Here's how the part is built. I have some questions about the finished solid (model axes, mm). A direction names the side the tool comes from. Coordinates: 2 decimals unless noted, no trailing zeros. Write each loop counter-clockwise with the first axis right and the second up, starting at its lowest first coordinate (ties: lowest second). Pieces come first, ordered by that corner, then holes. Notation, with made-up numbers: (-5, -33.75) -> (37, -33.75) arc R25 cw to (37, -12.75) -> close; hole circle Ø9 at (53, 67.5). An arc over 180 degrees is marked (long way). Put each result on its own line as item: value. Start each with the question number.
Item 1: For pin 1 (12 mm diameter, centred on x = -24, z = -40.5, fed in from +Y); pin 2 (5 mm diameter, centred on x = -10.5, z = -44.5, fed in from +Y); pin 3 (3 mm diameter, centred on y = -13, z = -85.5, fed in from +X); pin 4 (3.5 mm diameter, centred on x = 10.5, z = -44.5, fed in from +Y), each with a flat end and sliding along its axis, tell me the tip position at first contact or that it passes through.
Item 2: On a 3-axis mill with a long thin cutter (end or side, diameter ignored), from which of +Z, -Z, +X, -X, +Y, -Y can I reach the whole of each face in a straight line? I mean faces 1 (the face through (37, 20, -38)), 2 (the face through (0, -18, -52)), 3 (the face through (-50, 4.25, -20)), 4 (the face through (43.802, -2.095, -20.218)), 5 (the face through (-44.753, -0.121, -13.944)). Say none if no direction works.
Item 3: I want a section at C-C, the plane x = -47.5. List the corners of the cut face in (y, z) for me.
Item 4: I want a section at B-B, the plane x = -10.5. List the corners of the cut face in (y, z) for me.
Item 5: I want a section at D-D, the plane z = -126.5. List the corners of the cut face in (x, y) for me.
Item 6: I need wall thicknesses on line 1 (X direction, y = 0, z = -14.5); line 2 (X direction, y = 9, z = -44); line 3 (Z direction, x = -10.5, y = -5). Which ranges of each line are inside material? Lowest first, please. Write a range as [from, to].
Item 7: I want a section at A-A, the plane y = -13. List the corners of the cut face in (x, z) for me.
Item 8: If we mould it in two halves opening along Y, with no side actions, what happens to faces 6 (the face through (-36, 20, -38)), 7 (the face through (49, 0, -22.5)), 8 (the face through (37, -20, -38))? For each: released by +Y, released by -Y, zero draft, split by the parting line, or undercut.
from build123d import *

# Parameters (mm, degrees)
PAD_DEPTH       = 20
SKETCH003_R     = 2.2
HOLE_DEPTH      = 40.001
POCKET001_DEPTH = 4.5
SKETCH007_R     = 2.75
HOLE001_DEPTH   = 12
PAD001_DEPTH    = 101
SKETCH011_R     = 45
HOLE002_DEPTH   = 12
CHAMFER_SIZE    = 0.99
SKETCH009_W     = 35
SKETCH009_H     = 67.5
POCKET_DEPTH    = 2


with BuildPart() as part:
    # Sketch → Pad (new body, symmetric)
    with BuildSketch(Plane.XZ):
        with BuildLine():
            ThreePointArc((13.9194109071, -37.5), (29.6992968462, -26.794621976), (38.7298334621, -10))
            Line((38.7298334621, -10), (55, -10))
            Line((55, -10), (55, -45.8493649054))
            Line((0, -77.6036297108), (55, -45.8493649054))
            Line((-55, -45.8493649054), (0, -77.6036297108))
            Line((-55, -45.8493649054), (-55, -10))
            Line((-55, -10), (-38.7298334621, -10))
            ThreePointArc((-38.7298334621, -10), (-29.6992968462, -26.794621976), (-13.9194109071, -37.5))
            Line((-13.9194109071, -37.5), (13.9194109071, -37.5))
        make_face()
    extrude(amount=PAD_DEPTH, both=True)

    # Sketch003 → Hole (cut, through all)
    with BuildSketch(Plane.XZ.offset(20)):
        with Locations((-10.5, -44.5)):
            Circle(SKETCH003_R)
        with Locations((10.5, -44.5)):
            Circle(SKETCH003_R)
        with Locations((-10.5, -60.5)):
            Circle(SKETCH003_R)
        with Locations((10.5, -60.5)):
            Circle(SKETCH003_R)
    extrude(amount=-HOLE_DEPTH, mode=Mode.SUBTRACT)

    # Sketch006 → Pocket001 (cut)
    with BuildSketch(Plane(origin=(0, 0, -18), x_dir=(-1, 0, 0), z_dir=(0, 0, 1))):
        Polygon((55, 4.25), (45.0462616441, 4.25), (42.592523, 0), (45.0462616441, -4.25), (55, -4.25), align=None)
        Polygon((-55, 4.25), (-55, -4.25), (-45.0462616441, -4.25), (-42.592523, 0), (-45.0462616441, 4.25), align=None)
    extrude(amount=-POCKET001_DEPTH, mode=Mode.SUBTRACT)

    # Sketch007 (on Face5 of Pocket001) → Hole001 (cut)
    with BuildSketch(Plane(origin=(0, 0, -10), x_dir=(-1, 0, 0), z_dir=(0, 0, 1))):
        with Locations((47.5, 0)):
            Circle(SKETCH007_R)
        with Locations((-47.5, 0)):
            Circle(SKETCH007_R)
    extrude(amount=-HOLE001_DEPTH, mode=Mode.SUBTRACT)

    # Sketch010 (on Face10 of Hole001) → Pad001 (join)
    with BuildSketch(Plane(origin=(33.1033573777, 0, -57.3366968793), x_dir=(0.8660254038, 0, 0.5), z_dir=(0.5, 0, -0.8660254038))):
        Polygon((-38.8, 9), (-38.8, -9), (-26.8, -21), (-20.8, -21), (-2.8, -3), (-2.8, 3), (-20.8, 21), (-26.8, 21), align=None)
    extrude(amount=PAD001_DEPTH)

    # Sketch011 (on Face30 of Pad001) → Hole002 (cut)
    with BuildSketch(Plane(origin=(-33.6017856668, 0, -19.4), x_dir=(0.5, 0, -0.8660254038), z_dir=(-0.8660254038, 0, -0.5))):
        with Locations((117.5, 0)):
            Circle(SKETCH011_R)
    extrude(amount=-HOLE002_DEPTH, mode=Mode.SUBTRACT)

    # Chamfer
    chamfer_edges = [part.edges().sort_by_distance(p)[0] for p in [
        (9.460864, 20.5, -70.986697),
        (12.491953, 21, -69.236697),
        (15.523042, 20.5, -67.486697),
        (15.523042, -20.5, -67.486697),
        (12.491953, -21, -69.236697),
        (9.460864, -20.5, -70.986697),
    ]]
    chamfer(chamfer_edges, length=CHAMFER_SIZE)

    # Sketch009 → Pocket (cut)
    with BuildSketch(Plane(origin=(0, 20, 0), x_dir=(1, 0, 0), z_dir=(0, 1, 0))):
        with Locations((0, 33.75)):
            Rectangle(SKETCH009_W, SKETCH009_H)
    pocket = extrude(amount=-POCKET_DEPTH, mode=Mode.SUBTRACT)

    # Mirrored: Pocket across XZ
    add(pocket.mirror(Plane.XZ), mode=Mode.SUBTRACT)


solid = part.part
Calculated:
1. pin 1: stops at y = 20
1. pin 2: stops at y = 18
1. pin 3: stops at x = 36.52
1. pin 4: passes through
2. face 1: +Z, +X, -X, +Y
2. face 2: +Z, -Y
2. face 3: -X
2. face 4: +X
2. face 5: +Z
3. outline: (-20, -50.18) -> (20, -50.18) -> (20, -10) -> (2.75, -10) -> (2.75, -18) -> (4.25, -18) -> (4.25, -22.5) -> (-4.25, -22.5) -> (-4.25, -18) -> (-2.75, -18) -> (-2.75, -10) -> (-20, -10) -> close
4. outline: (-20, -71.54) -> (20, -71.54) -> (20, -67.5) -> (18, -67.5) -> (18, -62.7) -> (-18, -62.7) -> (-18, -67.5) -> (-20, -67.5) -> close; (-18, -58.3) -> (18, -58.3) -> (18, -46.7) -> (-18, -46.7) -> close; (-18, -42.3) -> (18, -42.3) -> (18, -37.5) -> (-18, -37.5) -> close
5. outline: (42.09, -21) -> (49.02, -21) -> (69.8, -3) -> (69.8, 3) -> (49.02, 21) -> (42.09, 21) -> close
6. line 1: x = [-55, -50.25], [-44.75, -37.28], [37.28, 44.75], [50.25, 55]
6. line 2: x = [-55, -12.64], [-8.36, 8.36], [12.64, 55]
6. line 3: z = [-71.54, -62.7], [-58.3, -46.7], [-42.3, -37.5]
7. outline: (-55, -45.85) -> (0, -77.6) -> (3.47, -75.6) -> (7.07, -81.85) -> (14, -77.85) -> (57.08, -152.47) -> (50.15, -156.47) -> (53.47, -162.21) -> (72.52, -151.21) -> (22.52, -64.6) -> (55, -45.85) -> (55, -10) -> (38.73, -10) arc R40 cw to (13.92, -37.5) -> (-13.92, -37.5) arc R40 cw to (-38.73, -10) -> (-55, -10) -> close; hole circle Ø4.4 at (-10.5, -60.5); hole circle Ø4.4 at (-10.5, -44.5); hole circle Ø4.4 at (10.5, -60.5); hole circle Ø4.4 at (10.5, -44.5)
8. face 6: released by +Y
8. face 7: undercut
8. face 8: released by -Y
